Verification items for the finished model (mm, model axes). Round coordinates to 2 decimals unless told otherwise and drop trailing zeros. Write each loop counter-clockwise with the first axis right and the second up, starting at its lowest first coordinate (ties: lowest second). Pieces come first, ordered by that corner, then holes. Notation, with made-up numbers: M 2,-39 L 60,-39 A8 ccw 60,-24 Z; hole C 28,33 d7. An arc over 180 degrees is marked long. One line per item, written item: value. Start each with the question number.
from build123d import *

# Parameters (mm, degrees)
BOSS_EXTRUDE1_DEPTH   = 1.6
ESBO_O1_R             = 1.6
CORTE_EXTRUS_O1_DEPTH = 10


with BuildPart() as part:
    # Sketch2 → Boss-Extrude1 (new body)
    with BuildSketch(Plane(origin=(0, 0, 0), x_dir=(1, 0, 0), z_dir=(0, 1, 0))):
        Polygon((50.8, -22.47), (50.8, 11.586871141), (48.2, 14.186871141), (48.2, 24.07), (45.6, 26.67), (-50.8, 26.67), (-50.8, -26.67), (48.2, -26.67), (48.2, -25.07), align=None)
    extrude(amount=BOSS_EXTRUDE1_DEPTH)

    # Esboço1 → Corte-extrusão1 (cut)
    with BuildSketch(Plane(origin=(0, 1.6, 0), x_dir=(1, 0, 0), z_dir=(0, 1, 0))):
        with Locations(Location((-35.5, 24.17, 0), (0, 0, 270))):
            Circle(ESBO_O1_R)
        with Locations(Location((-36.8, -24.17, 0), (0, 0, 270))):
            Circle(ESBO_O1_R)
        with Locations(Location((39.4, 24.17, 0), (0, 0, 270))):
            Circle(ESBO_O1_R)
        with Locations(Location((45.7, -24.17, 0), (0, 0, 270))):
            Circle(ESBO_O1_R)
        with Locations(Location((15.3, 8.83, 0), (0, 0, 270))):
            Circle(ESBO_O1_R)
        with Locations(Location((15.3, -19.07, 0), (0, 0, 270))):
            Circle(ESBO_O1_R)
    extrude(amount=-CORTE_EXTRUS_O1_DEPTH, mode=Mode.SUBTRACT)


solid = part.part
1) Thickness scan on line 1 (X direction, y = 0.2, z = 23.5); line 2 (X direction, y = 0.7, z = 19.07); line 3 (X direction, y = 0.7, z = -24.17). Record the ranges inside material, lowest first.
2) Cross-section at D-D (z = -15.5). Record the boundary of the cut face in (x, y), then the cut area to 3 significant figures.
3) Cross-section at A-A (z = -8.83). Record the boundary of the cut face in (x, y).
4) Cross-section at C-C (y = 0.75). Record the boundary of the cut face in (x, z).
5) Gauge pin test, flat ends, axial feed: pin 1 Ø1.9 at (x, z) = (39.4, -24.17) entering from -Y; pin 2 Ø0.5 at (y, z) = (1, -21) entering from +X. Record the tip position at first contact, or that the pin passes through.
6) Mould release check, pull along X, two halves, no side actions. Record for faces 1 (the cylindrical face through (39.47, 0.81, -25.77)), 2 (the flat face through (-1, 1.6, 0)), 3 (the flat face through (46.92, 0.79, -25.35)): pulls with the +X half, pulls with the -X half, needs draft (parallel to the pull), parting line crosses it, or undercut.
7) Cross-section at B-B (x = 15.3). Record the boundary of the cut face in (y, z), then the cut area to 3 significant figures.
Results below:
1. line 1: x = -50.8 to -38.25, -35.35 to 44.25, 47.15 to 49.77
1. line 2: x = -50.8 to 13.7, 16.9 to 50.8
1. line 3: x = -50.8 to -37.1, -33.9 to 37.8, 41 to 48.1
2. outline: M -50.8,0 L 48.2,0 L 48.2,1.6 L -50.8,1.6 Z
2. area: 158 mm²
3. outline: M -50.8,0 L 13.7,0 L 13.7,1.6 L -50.8,1.6 Z; M 16.9,0 L 50.8,0 L 50.8,1.6 L 16.9,1.6 Z
4. outline: M -50.8,-26.67 L 45.6,-26.67 L 48.2,-24.07 L 48.2,-14.19 L 50.8,-11.59 L 50.8,22.47 L 48.2,25.07 L 48.2,26.67 L -50.8,26.67 Z; hole C -36.8,24.17 d3.2; hole C -35.5,-24.17 d3.2; hole C 15.3,-8.83 d3.2; hole C 15.3,19.07 d3.2; hole C 39.4,-24.17 d3.2; hole C 45.7,24.17 d3.2
5. pin 1: passes through
5. pin 2: stops at x = 48.2
6. face 1: undercut
6. face 2: needs draft
6. face 3: pulls with the +X half
7. outline: M 0,-26.67 L 1.6,-26.67 L 1.6,-10.43 L 0,-10.43 Z; M 0,-7.23 L 1.6,-7.23 L 1.6,17.47 L 0,17.47 Z; M 0,20.67 L 1.6,20.67 L 1.6,26.67 L 0,26.67 Z
7. area: 75.1 mm²
